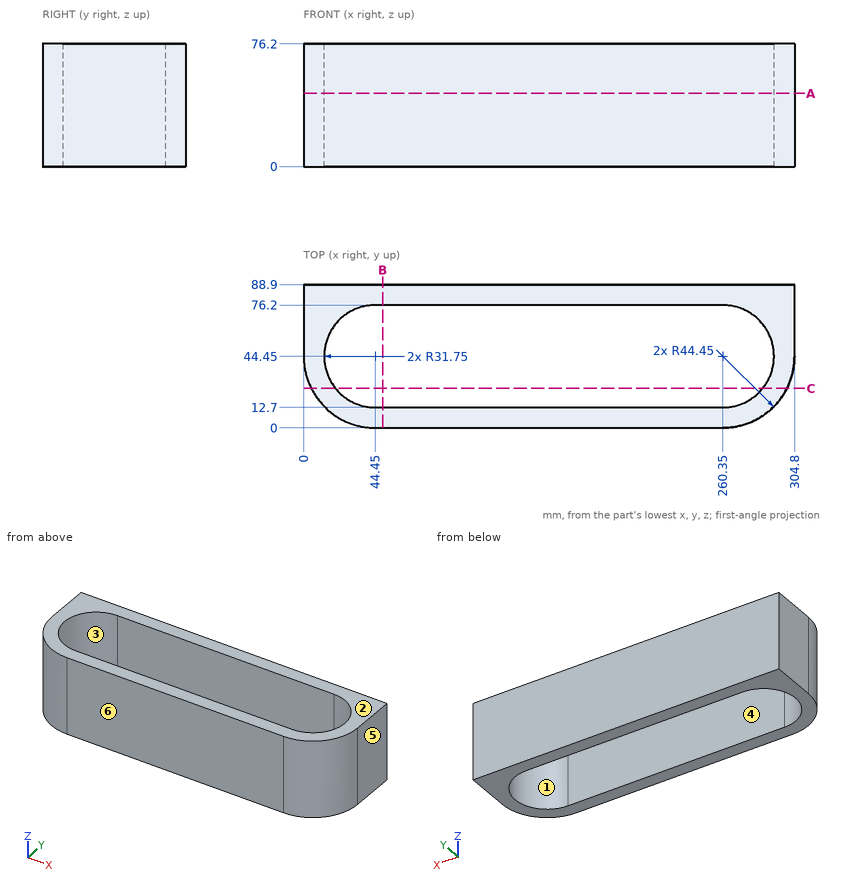
Source: three-view drawing plus pictorial views. Frame: mm from the lowest corner of the part. A direction names the side the tool comes from. Round coordinates to 2 decimals unless told otherwise and drop trailing zeros. Loops run counter-clockwise (first coordinate to the right, second up) from the corner with the lowest first, then second, coordinate; pieces in that order, holes last.
Q1. Ray query, line 1 (Y direction, x = 178, z = 34.5); line 2 (X direction, y = 43, z = 60); line 3 (Y direction, x = 269.5, z = 49). Return the intervals inside material, ascending.
Q2. Access query for the marked faces 1 and 2. Directions: +Z, -Z, +X, -X, +Y, -Y. A direction counts if a zero-diameter tool reaches every point of the face in a straight line with its end or side. Return the directions, or none.
Q3. Section A-A, the plane z = 45.5. Return loops of the section in (x, y).
Q4. Section B-B, the plane x = 49. Return loops of the section in (y, z).
Q5. First-contact query: P1, Ø12, axis at x = 133.5, z = 54.5, coming from the -Y side. Flat tip, straight axial feed; report the tip coordinate or a pass-through.
Q6. Mould query, pull axis X, two halves, no side actions, for the marked faces 3, 4, 5 and 6. Classes: pulls with the +X half, pulls with the -X half, needs draft (parallel to the pull), parting line crosses it, or undercut.
Q7. Section C-C, the plane y = 24.5. Return loops of the section in (x, z).
Solutions:
1. line 1: y = 0 to 12.7, 76.2 to 88.9
1. line 2: x = 0.02 to 12.73, 292.07 to 304.78
1. line 3: y = 0.95 to 14.05, 74.85 to 88.9
2. face 1: +Z, -Z
2. face 2: +Z, +X, -X, +Y, -Y
3. outline: (0, 44.45) arc R44.45 ccw to (44.45, 0) - (260.35, 0) arc R44.45 ccw to (304.8, 44.45) - (304.8, 88.9) - (0, 88.9) - close; hole (44.45, 12.7) - (260.35, 12.7) arc R31.75 ccw to (260.35, 76.2) - (44.45, 76.2) arc R31.75 ccw to start
4. outline: (0, 0) - (12.7, 0) - (12.7, 76.2) - (0, 76.2) - close; (76.2, 0) - (88.9, 0) - (88.9, 76.2) - (76.2, 76.2) - close
5. P1: stops at y = 0
6. face 3: undercut
6. face 4: undercut
6. face 5: pulls with the +X half
6. face 6: needs draft
7. outline: (4.73, 0) - (19.75, 0) - (19.75, 76.2) - (4.73, 76.2) - close; (285.05, 0) - (300.07, 0) - (300.07, 76.2) - (285.05, 76.2) - close
